Verification items for this drawing (mm, ordinates from the low corner). A direction names the side the tool comes from. Round coordinates to 2 decimals unless told otherwise and drop trailing zeros. Loops run counter-clockwise (first coordinate to the right, second up) from the corner with the lowest first, then second, coordinate; pieces in that order, holes last. Notation, with made-up numbers: (-39.5, -17.75) - (3.5, -17.75) arc R26 cw to (3.5, 10.25) - close; hole circle Ø6 at (43.25, 57.25). An arc over 180 degrees is marked (long way). Answer in a Markdown table with one row per item. Add a question column.
(1) Mould release check, pull along Z, two halves, no side actions. Record for the marked faces 4, 5 and 6: +Z half, -Z half, draft (parallel to the pull), parting line (faces both ways), or undercut.
(2) Cross-section at D-D on z = 5.75. Enter the section's corners in (x, y).
(3) Cross-section at A-A on x = 9.5. Enter the section's corners in (y, z).
(4) Cross-section at B-B on z = 9.5. Enter the section's corners in (x, y), then the cut area to 3 significant figures.
(5) Access from +Z, -Z, +X, -X, +Y, -Y to the whole of each face (thin tool, end or side, straight path). Record for the marked faces 1, 2 and 3.
(6) Gauge pin test, flat ends, axial feed: pin 1 (2 mm diameter, centred on y = 1.5, z = 2.5, fed in from +X); pin 2 (1.5 mm diameter, centred on y = 1.5, z = 8, fed in from -X); pin 3 (1.5 mm diameter, centred on x = 5.5, y = 5.5, fed in from +Z). Record the tip position at first contact, or that the pin passes through.
(7) Cross-section at C-C on y = 1.4. Enter the section's corners in (x, z), then the cut area to 3 significant figures.
(8) Thickness scan on line 1 along Z through (x, y) = (9.5, 5.7); line 2 along Y through (x, z) = (16, 10.5); line 3 along Z through (x, y) = (9, 3.2). Record the ranges inside material, lowest first.
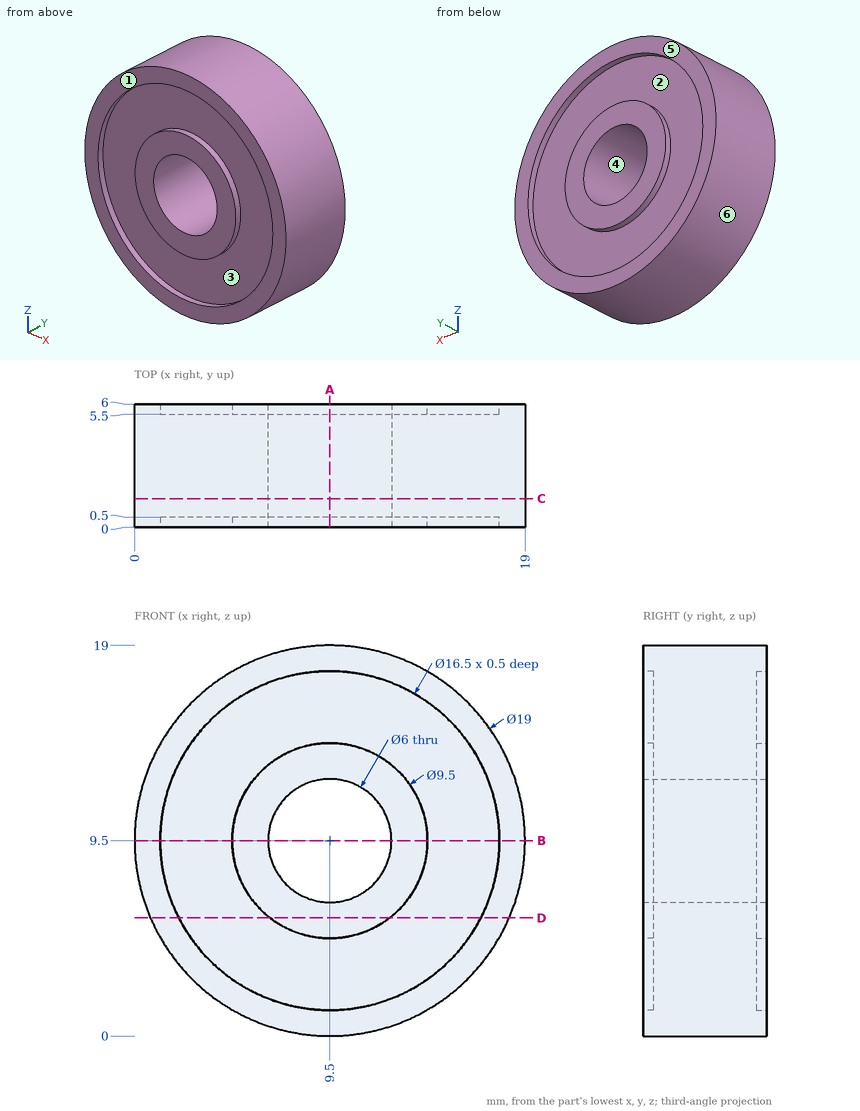
Answers:
| question | item | result |
|---|---|---|
| 1 | face 4 | undercut |
| 1 | face 5 | draft |
| 1 | face 6 | parting line |
| 2 | outline | (0.77, 0) - (2.15, 0) - (2.15, 0.5) - (6.58, 0.5) - (6.58, 0) - (12.42, 0) - (12.42, 0.5) - (16.85, 0.5) - (16.85, 0) - (18.23, 0) - (18.23, 6) - (16.85, 6) - (16.85, 5.5) - (12.42, 5.5) - (12.42, 6) - (6.58, 6) - (6.58, 5.5) - (2.15, 5.5) - (2.15, 6) - (0.77, 6) - close |
| 3 | outline | (0, 0) - (6, 0) - (6, 1.25) - (5.5, 1.25) - (5.5, 4.75) - (6, 4.75) - (6, 6.5) - (0, 6.5) - (0, 4.75) - (0.5, 4.75) - (0.5, 1.25) - (0, 1.25) - close; (0, 12.5) - (6, 12.5) - (6, 14.25) - (5.5, 14.25) - (5.5, 17.75) - (6, 17.75) - (6, 19) - (0, 19) - (0, 17.75) - (0.5, 17.75) - (0.5, 14.25) - (0, 14.25) - close |
| 4 | outline | (0, 0) - (1.25, 0) - (1.25, 0.5) - (4.75, 0.5) - (4.75, 0) - (6.5, 0) - (6.5, 6) - (4.75, 6) - (4.75, 5.5) - (1.25, 5.5) - (1.25, 6) - (0, 6) - close; (12.5, 0) - (14.25, 0) - (14.25, 0.5) - (17.75, 0.5) - (17.75, 0) - (19, 0) - (19, 6) - (17.75, 6) - (17.75, 5.5) - (14.25, 5.5) - (14.25, 6) - (12.5, 6) - close |
| 4 | area | 71.0 mm^2 |
| 5 | face 1 | +Z, -Z, +X, -X, -Y |
| 5 | face 2 | +Y |
| 5 | face 3 | -Y |
| 6 | pin 1 | stops at x = 16.87 |
| 6 | pin 2 | stops at x = 0.03 |
| 6 | pin 3 | stops at z = 18.43 |
| 7 | outline | circle Ø19 at (9.5, 9.5); hole circle Ø6 at (9.5, 9.5) |
| 7 | area | 255 mm^2 |
| 8 | line 1 | z = 0 to 1.25, 4.75 to 6.5, 12.5 to 14.25, 17.75 to 19 |
| 8 | line 2 | y = 0.5 to 5.5 |
| 8 | line 3 | z = 0.01 to 6.54, 12.46 to 18.99 |
